```python
from build123d import *

# Parameters (mm, degrees)
SKETCH1_W                       = 58.039
SKETCH1_H                       = 29.464
BOSS_EXTRUDE1_DEPTH             = 4.826
F_25_0_1495_DIAMETER_HOLE1_D    = 3.7846
SKETCH4_W                       = 32.258
SKETCH4_H                       = 13.97
BOSS_EXTRUDE2_DEPTH             = 18.034
FILLET1_R                       = 2.54
FILLET2_R                       = 1.27
BOSS_EXTRUDE3_DEPTH             = 7.6962
BOSS_EXTRUDE3_DEPTH_BACK        = 30.5562
BOSS_EXTRUDE4_REACH             = 46.641
BOSS_EXTRUDE4_DIRECTION_2_REACH = 46.641


with BuildPart() as part:
    # Sketch1 → Boss-Extrude1 (new body)
    with BuildSketch(Plane.XY):
        Rectangle(SKETCH1_W, SKETCH1_H)
    extrude(amount=BOSS_EXTRUDE1_DEPTH)

    # #25 (0.1495) Diameter Hole1 (through all)
    with Locations(Plane.XY.offset(4.826)):
        with Locations((-24.5999, 10.16), (24.5999, 10.16), (24.5999, -10.16), (-24.5999, -10.16)):
            Hole(F_25_0_1495_DIAMETER_HOLE1_D / 2)

    # Sketch4 → Boss-Extrude2 (add)
    with BuildSketch(Plane.XY.offset(4.826)):
        Rectangle(SKETCH4_W, SKETCH4_H)
    extrude(amount=BOSS_EXTRUDE2_DEPTH)

    # Fillet1
    fillet1_edges = [part.edges().sort_by_distance(p)[0] for p in [
        (29.0195, -14.732, 2.413),
        (-29.0195, -14.732, 2.413),
        (-29.0195, 14.732, 2.413),
        (29.0195, 14.732, 2.413),
    ]]
    fillet(fillet1_edges, radius=FILLET1_R)

    # Fillet2
    fillet2_edges = [part.edges().sort_by_distance(p)[0] for p in [
        (16.129, -6.985, 13.843),
        (16.129, 6.985, 13.843),
        (-16.129, 6.985, 13.843),
        (-16.129, -6.985, 13.843),
    ]]
    fillet(fillet2_edges, radius=FILLET2_R)

    # Sketch5 → Boss-Extrude3 (add, two sides: drawn at the far end of the back side and taken through both)
    with BuildSketch(Plane.XY.offset(22.86).offset(-BOSS_EXTRUDE3_DEPTH_BACK)):
        with BuildLine():
            Line((8.108705846, 2.421066814), (7.177135142, -2.862133186))
            ThreePointArc((7.177135142, -2.862133186), (6.74276956, -3.614476443), (5.926429296, -3.9116))
            Line((5.926429296, -3.9116), (-5.926429296, -3.9116))
            ThreePointArc((-5.926429296, -3.9116), (-6.74276956, -3.614476443), (-7.177135142, -2.862133186))
            Line((-7.177135142, -2.862133186), (-8.108705846, 2.421066814))
            ThreePointArc((-8.108705846, 2.421066814), (-7.830876443, 3.457940264), (-6.858, 3.9116))
            Line((-6.858, 3.9116), (6.858, 3.9116))
            ThreePointArc((6.858, 3.9116), (7.830876443, 3.457940264), (8.108705846, 2.421066814))
        make_face()
    extrude(amount=BOSS_EXTRUDE3_DEPTH + BOSS_EXTRUDE3_DEPTH_BACK)

    # Boss-Extrude4: up to this face of the body (flat: up to its plane)
    boss_extrude4_end = Plane(part.part.faces().sort_by_distance((0, 0.101689946, 30.5562))[0])
    # Sketch6 → Boss-Extrude4 (add, up to the picked face)
    with BuildSketch(Plane.XY.offset(22.86), mode=Mode.PRIVATE) as boss_extrude4_sk1:
        Polygon((12.1285, -3.666174209), (15.3035, -1.833087105), (15.3035, 1.833087105), (12.1285, 3.666174209), (8.9535, 1.833087105), (8.9535, -1.833087105), align=None)
    boss_extrude4_tool1 = split(extrude(boss_extrude4_sk1.sketch, amount=BOSS_EXTRUDE4_REACH, mode=Mode.PRIVATE), bisect_by=boss_extrude4_end, keep=Keep.BOTH, mode=Mode.PRIVATE)
    # Sketch6 → Boss-Extrude4 (add, up to the picked face)
    with BuildSketch(Plane.XY.offset(22.86), mode=Mode.PRIVATE) as boss_extrude4_sk2:
        Polygon((-12.1285, -3.666174209), (-8.9535, -1.833087105), (-8.9535, 1.833087105), (-12.1285, 3.666174209), (-15.3035, 1.833087105), (-15.3035, -1.833087105), align=None)
    boss_extrude4_tool2 = split(extrude(boss_extrude4_sk2.sketch, amount=BOSS_EXTRUDE4_REACH, mode=Mode.PRIVATE), bisect_by=boss_extrude4_end, keep=Keep.BOTH, mode=Mode.PRIVATE)
    add(boss_extrude4_tool1.solids().sort_by(Axis((12.1285, 0, 22.86), (0, 0, 1)))[0])
    add(boss_extrude4_tool2.solids().sort_by(Axis((-12.1285, 0, 22.86), (0, 0, 1)))[0])

    # Boss-Extrude4 direction 2: up to this face of the body (flat: up to its plane)
    boss_extrude4_direction_2_end = Plane(part.part.faces().sort_by_distance((0, 0.101689946, -7.6962))[0])
    # Sketch6 → Boss-Extrude4 direction 2 (add, up to the picked face)
    with BuildSketch(Plane.XY.offset(22.86), mode=Mode.PRIVATE) as boss_extrude4_direction_2_sk1:
        Polygon((12.1285, -3.666174209), (15.3035, -1.833087105), (15.3035, 1.833087105), (12.1285, 3.666174209), (8.9535, 1.833087105), (8.9535, -1.833087105), align=None)
    boss_extrude4_direction_2_tool1 = split(extrude(boss_extrude4_direction_2_sk1.sketch, amount=-BOSS_EXTRUDE4_DIRECTION_2_REACH, mode=Mode.PRIVATE), bisect_by=boss_extrude4_direction_2_end, keep=Keep.BOTH, mode=Mode.PRIVATE)
    # Sketch6 → Boss-Extrude4 direction 2 (add, up to the picked face)
    with BuildSketch(Plane.XY.offset(22.86), mode=Mode.PRIVATE) as boss_extrude4_direction_2_sk2:
        Polygon((-12.1285, -3.666174209), (-8.9535, -1.833087105), (-8.9535, 1.833087105), (-12.1285, 3.666174209), (-15.3035, 1.833087105), (-15.3035, -1.833087105), align=None)
    boss_extrude4_direction_2_tool2 = split(extrude(boss_extrude4_direction_2_sk2.sketch, amount=-BOSS_EXTRUDE4_DIRECTION_2_REACH, mode=Mode.PRIVATE), bisect_by=boss_extrude4_direction_2_end, keep=Keep.BOTH, mode=Mode.PRIVATE)
    add(boss_extrude4_direction_2_tool1.solids().sort_by(Axis((12.1285, 0, 22.86), (0, 0, -1)))[0])
    add(boss_extrude4_direction_2_tool2.solids().sort_by(Axis((-12.1285, 0, 22.86), (0, 0, -1)))[0])


solid = part.part
```
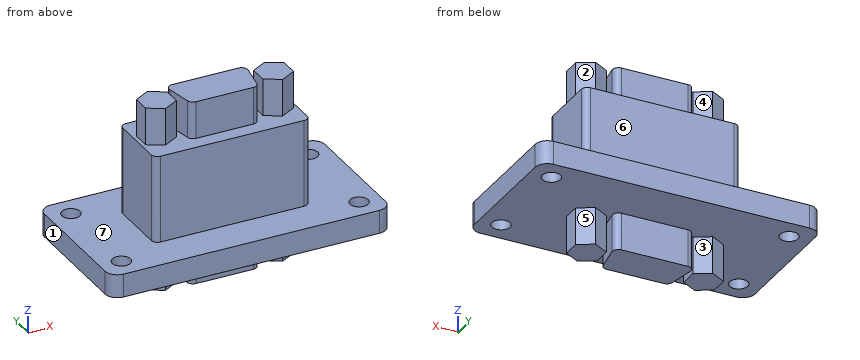
CAD build for the part. Positions are in the model's coordinates, mm. Face numbers are marked on the shaded views. A direction names the side the tool comes from. Round coordinates to 2 decimals unless told otherwise and drop trailing zeros. Write each loop counter-clockwise with the first axis right and the second up, starting at its lowest first coordinate (ties: lowest second). Pieces come first, ordered by that corner, then holes. Notation, with made-up numbers: (12.5, 50.5) - (35.5, 50.5) arc R19 ccw to (35.5, 80.5) - close; hole circle Ø4 at (21, 21). An arc over 180 degrees is marked (long way). Write item = value, one per line. Start each with the question number.
Q1. Mould opens along X. For the marked faces 1, 2, 3 and 4 say: pulls with the +X half, pulls with the -X half, needs draft (parallel to the pull), parting line crosses it, or undercut.
Q2. Band-saw the part on B-B (z = 28). Give the cut face in (x, y), then the cut area to 3 significant figures.
Q3. Band-saw the part on A-A (y = -10.16). Give the cut face in (x, z).
Q4. Band-saw the part on D-D (x = 22). Give the cut face in (y, z), then the cut area to 3 significant figures.
Q5. Drop flat-ended pins along their axis: pin 1 (4 mm diameter, centred on x = 2, z = -5, fed in from -Y); pin 2 (20 mm diameter, centred on x = 6.5, z = 11.5, fed in from -Y); pin 3 (4 mm diameter, centred on y = -0.5, z = 26.5, fed in from -X); pin 4 (1.1 mm diameter, centred on y = -0.5, z = -4, fed in from +X). Give the stop position or say it passes through.
Q6. Which spindle directions (+Z, -Z, +X, -X, +Y, -Y) get a long thin tool onto all of the face, cutting with end or side? Do the marked faces 5, 6 and 7. Say none if no direction does.
Q7. Probe L1, parallel to Z at x = 13, y = 9.5; L2, parallel to Y at x = -26, z = 4.5; L3, parallel to X at y = -5.5, z = 13. List the from-to ranges inside material, lowest first. Write a range as from..to.
Q8. Band-saw the part on C-C (z = 2). Give the cut face in (x, y), then the cut area to 3 significant figures.
Answers below:
q1.face_1 = pulls with the -X half
q1.face_2 = pulls with the +X half
q1.face_3 = undercut
q1.face_4 = undercut
q2.outline = (-15.3, -1.83) - (-12.13, -3.67) - (-8.95, -1.83) - (-8.95, 1.83) - (-12.13, 3.67) - (-15.3, 1.83) - close; (-8.11, 2.42) - (-7.18, -2.86) arc R1.27 ccw to (-5.93, -3.91) - (5.93, -3.91) arc R1.27 ccw to (7.18, -2.86) - (8.11, 2.42) arc R1.27 ccw to (6.86, 3.91) - (-6.86, 3.91) arc R1.27 ccw to start; (8.95, -1.83) - (12.13, -3.67) - (15.3, -1.83) - (15.3, 1.83) - (12.13, 3.67) - (8.95, 1.83) - close
q2.area = 189 mm2
q3.outline = (-29.02, 0) - (-26.49, 0) - (-26.49, 4.83) - (-29.02, 4.83) - close; (-22.71, 0) - (22.71, 0) - (22.71, 4.83) - (-22.71, 4.83) - close; (26.49, 0) - (29.02, 0) - (29.02, 4.83) - (26.49, 4.83) - close
q4.outline = (-14.73, 0) - (14.73, 0) - (14.73, 4.83) - (-14.73, 4.83) - close
q4.area = 142 mm2
q5.pin_1 = -3.91
q5.pin_2 = -14.73
q5.pin_3 = -15.3
q5.pin_4 = 15.3
q6.face_5 = -Z, +X, +Y
q6.face_6 = +Z, +X, -X, +Y
q6.face_7 = +Z
q7.L1 = 0..4.83
q7.L2 = -14.73..-11.43, -8.89..8.89, 11.43..14.73
q7.L3 = -16.13..16.13
q8.outline = (-29.02, -12.19) arc R2.54 ccw to (-26.48, -14.73) - (26.48, -14.73) arc R2.54 ccw to (29.02, -12.19) - (29.02, 12.19) arc R2.54 ccw to (26.48, 14.73) - (-26.48, 14.73) arc R2.54 ccw to (-29.02, 12.19) - close; hole circle Ø3.78 at (-24.6, -10.16); hole circle Ø3.78 at (-24.6, 10.16); hole circle Ø3.78 at (24.6, -10.16); hole circle Ø3.78 at (24.6, 10.16)
q8.area = 1,660 mm2
